from build123d import *

# Parameters (mm, degrees)
BOSS_EXTRUDE1_DEPTH = 6.35
SKETCH2_R           = 1.700000029
CUT_EXTRUDE1_DEPTH  = 61.705405925


with BuildPart() as part:
    # Sketch1 → Boss-Extrude1 (new body)
    with BuildSketch(Plane.XY):
        with BuildLine():
            Line((-16.5, 0), (-25.2499952, 0))
            Line((-25.2499952, 0), (-25.2499952, -20.32))
            Line((-25.2499952, -20.32), (-28.4249952, -20.32))
            Line((-28.4249952, -20.32), (-28.4249952, 3.350143749))
            Line((-28.4249952, 3.350143749), (-18.194134683, 3.350143749))
            ThreePointArc((-18.194134683, 3.350143749), (0, 18.5), (18.194134683, 3.350143749))
            Line((18.194134683, 3.350143749), (28.4249952, 3.350143749))
            Line((28.4249952, 3.350143749), (28.4249952, -20.32))
            Line((28.4249952, -20.32), (25.2499952, -20.32))
            Line((25.2499952, -20.32), (25.2499952, 0))
            Line((25.2499952, 0), (16.5, 0))
            ThreePointArc((16.5, 0), (0, 16.5), (-16.5, 0))
        make_face()
    extrude(amount=BOSS_EXTRUDE1_DEPTH)

    # Sketch2 → Cut-Extrude1 (cut, through all)
    with BuildSketch(Plane(origin=(28.4249952, 0, 0), x_dir=(0, 0, -1), z_dir=(1, 0, 0))):
        with Locations(Location((-3.175, -15.587842251, 0), (0, 0, 90))):
            Circle(SKETCH2_R)
    extrude(amount=-CUT_EXTRUDE1_DEPTH, mode=Mode.SUBTRACT)


solid = part.part
Could you check a few things on this model? Use its own coordinates, in mm. A direction names the side the tool comes from. Coordinates: 2 decimals unless noted, no trailing zeros. Order: outer loops, then holes, each group sorted by start corner. A loop starts at its lowest first (then second) coordinate and runs counter-clockwise, first axis right, second up.
Q1. Suppose I cut it at B-B on z = 4.25. Please give me the cut outline in (x, y) (3 decimals), and give its area (3 significant figures).
Q2. Suppose I cut it at C-C on x = 0. Please give me the cut outline in (y, z).
Q3. Please list where these lines run through material, in increasing order: L1, parallel to X at y = -14.5, z = 4.75 (3 decimals); L2, parallel to Y at x = 0.5, z = 6; L3, parallel to X at y = 10, z = 5.25.
Q4. Suppose I cut it at A-A on y = -1. Please give me the cut outline in (x, z) (3 decimals).
Q5. Thinking about a two-plate mould opening in Z: for faces 4 (the flat face through (25.25, -10, 3)), 5 (the flat face through (17, 1, 6.35)), 6 (the cylindrical face through (26.86, -14.02, 2.52)), 7 (the cylindrical face through (-26.82, -14.02, 2.52)), which applies, released by +Z, released by -Z, zero draft, split by the parting line, or undercut?
Q6. Suppose I cut it at D-D on y = 13.5. Please give me the cut outline in (x, z).
Q7. Will these pins go through, and if not, where does the flat tip stop? pin 1 (1 mm diameter, centred on x = 14, z = 2.5, fed in from +Y); pin 2 (3 mm diameter, centred on x = -5.5, z = 5.5, fed in from +Y); pin 3 (1 mm diameter, centred on y = 3.5, z = 4, fed in from -X) (3 decimals); pin 4 (1.9 mm diameter, centred on x = -26, z = 3.5, fed in from +Y).
Q8. Which directions (+Z, -Z, +X, -X, +Y, -Y) give clear straight access to the entire face, cutting with the end or side of a thin tool? Please do faces 1 (the flat face through (23, 3.35, 3)), 2 (the flat face through (-23, 3.35, 3)), 3 (the flat face through (21, 0, 3)).
Answer:
1. outline: (-28.425, -20.32) - (-25.25, -20.32) - (-25.25, -16.905) - (-28.425, -16.905) - close; (-28.425, -14.271) - (-25.25, -14.271) - (-25.25, 0) - (-16.5, 0) arc R16.5 cw to (16.5, 0) - (25.25, 0) - (25.25, -14.271) - (28.425, -14.271) - (28.425, 3.35) - (18.194, 3.35) arc R18.5 ccw to (-18.194, 3.35) - (-28.425, 3.35) - close; (25.25, -20.32) - (28.425, -20.32) - (28.425, -16.905) - (25.25, -16.905) - close
1. area: 289 mm2
2. outline: (16.5, 0) - (18.5, 0) - (18.5, 6.35) - (16.5, 6.35) - close
3. L1: x = -28.425 to -25.25, 25.25 to 28.425
3. L2: y = 16.49 to 18.49
3. L3: x = -15.56 to -13.12, 13.12 to 15.56
4. outline: (-28.425, 0) - (-25.25, 0) - (-25.25, 6.35) - (-28.425, 6.35) - close; (25.25, 0) - (28.425, 0) - (28.425, 6.35) - (25.25, 6.35) - close
5. face 4: zero draft
5. face 5: released by +Z
5. face 6: undercut
5. face 7: undercut
6. outline: (-12.65, 0) - (-9.49, 0) - (-9.49, 6.35) - (-12.65, 6.35) - close; (9.49, 0) - (12.65, 0) - (12.65, 6.35) - (9.49, 6.35) - close
7. pin 1: stops at y = 12.65
7. pin 2: stops at y = 18.06
7. pin 3: stops at x = -28.425
7. pin 4: stops at y = 3.35
8. face 1: +Z, -Z, +X, +Y
8. face 2: +Z, -Z, -X, +Y
8. face 3: +Z, -Z, -Y
